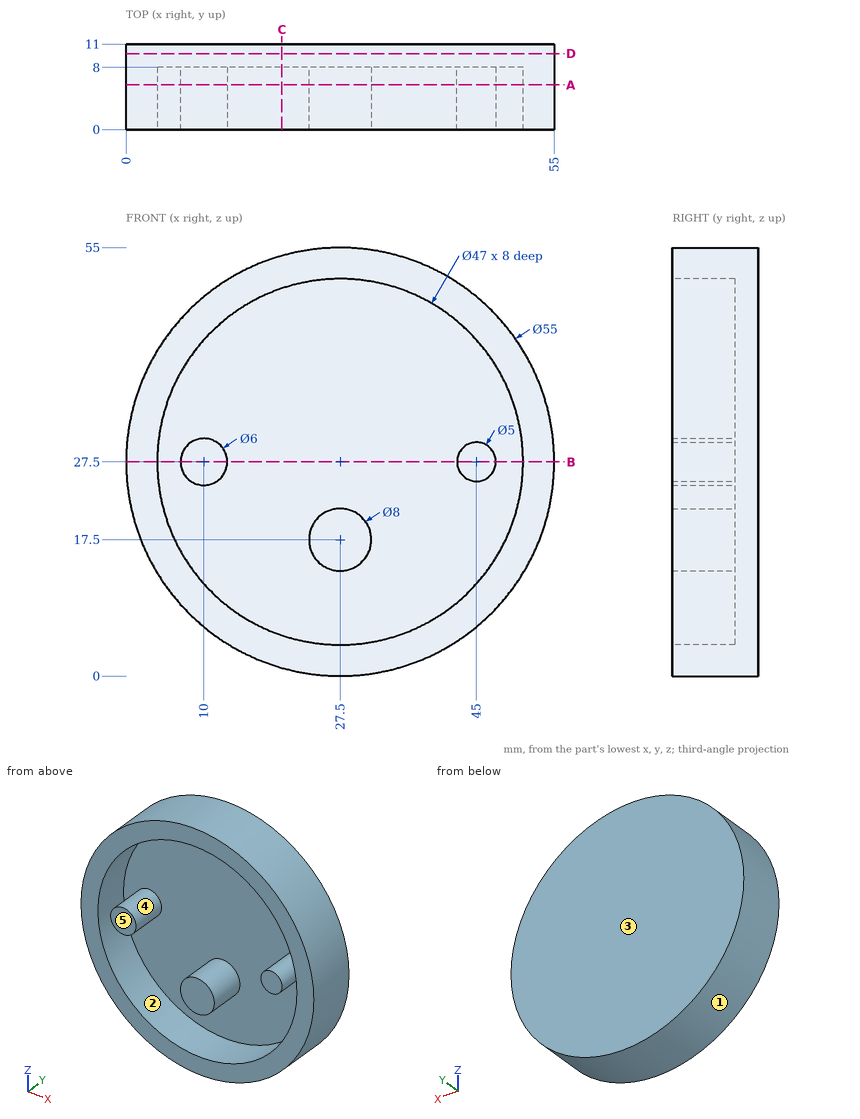
Drawing for the job (mm, zero at the part's lowest x, y, z). A direction names the side the tool comes from. Round coordinates to 2 decimals unless told otherwise and drop trailing zeros. Write each loop counter-clockwise with the first axis right and the second up, starting at its lowest first coordinate (ties: lowest second). Pieces come first, ordered by that corner, then holes. Notation, with made-up numbers: (27, -35.5) - (50, -35.5) arc R27 cw to (50, -2.5) - close; hole circle Ø9 at (3.5, 70.5). An arc over 180 degrees is marked (long way). Write item = value, one per line. Start each with the question number.
Q1. Which spindle directions (+Z, -Z, +X, -X, +Y, -Y) get a long thin tool onto all of the face, cutting with end or side? Do the marked faces 4 and 5. Say none if no direction does.
Q2. Drop flat-ended pins along their axis: pin 1 (4 mm diameter, centred on y = 5, z = 41.5, fed in from -X); pin 2 (1.5 mm diameter, centred on x = 26, y = 3.5, fed in from +Z); pin 3 (1 mm diameter, centred on x = 30, z = 13, fed in from -Y). Give the stop position or say it passes through.
Q3. Probe L1, parallel to Z at x = 27.5, y = 1.5; L2, parallel to Y at x = 49, z = 29; L3, parallel to X at y = 1.75, z = 7.5. List the from-to ranges inside material, lowest first. Write a range as from..to.
Q4. Band-saw the part on D-D (y = 9.75). Give the cut face in (x, z), then the cut area to 3 significant figures.
Q5. Band-saw the part on B-B (z = 27.5). Give the cut face in (x, y).
Q6. Mould opens along Z. For the marked faces 1, 2 and 3 say: pulls with the +Z half, pulls with the -Z half, needs draft (parallel to the pull), parting line crosses it, or undercut.
Q7. Band-saw the part on C-C (x = 20). Give the cut face in (y, z), then the cut area to 3 significant figures.
Q8. Band-saw the part on A-A (y = 5.75). Give the cut face in (x, z), then the cut area to 3 significant figures.
Answers below:
q1.face_4 = -Y
q1.face_5 = +Z, -Z, +X, -X, -Y
q2.pin_1 = 2.76
q2.pin_2 = 54.99
q2.pin_3 = 8
q3.L1 = 0..4, 13.5..21.5, 51..55
q3.L2 = 8..11
q3.L3 = 8.63..15.16, 39.84..46.37
q4.outline = circle Ø55 at (27.5, 27.5)
q4.area = 2,380 mm2
q5.outline = (0, 0) - (4, 0) - (4, 8) - (7, 8) - (7, 0) - (13, 0) - (13, 8) - (42.5, 8) - (42.5, 0) - (47.5, 0) - (47.5, 8) - (51, 8) - (51, 0) - (55, 0) - (55, 11) - (0, 11) - close
q6.face_1 = parting line crosses it
q6.face_2 = undercut
q6.face_3 = needs draft
q7.outline = (0, 1.04) - (11, 1.04) - (11, 53.96) - (0, 53.96) - (0, 49.77) - (8, 49.77) - (8, 5.23) - (0, 5.23) - close
q7.area = 226 mm2
q8.outline = circle Ø55 at (27.5, 27.5); circle Ø6 at (10, 27.5); circle Ø8 at (27.5, 17.5); circle Ø5 at (45, 27.5); hole circle Ø47 at (27.5, 27.5)
q8.area = 739 mm2
